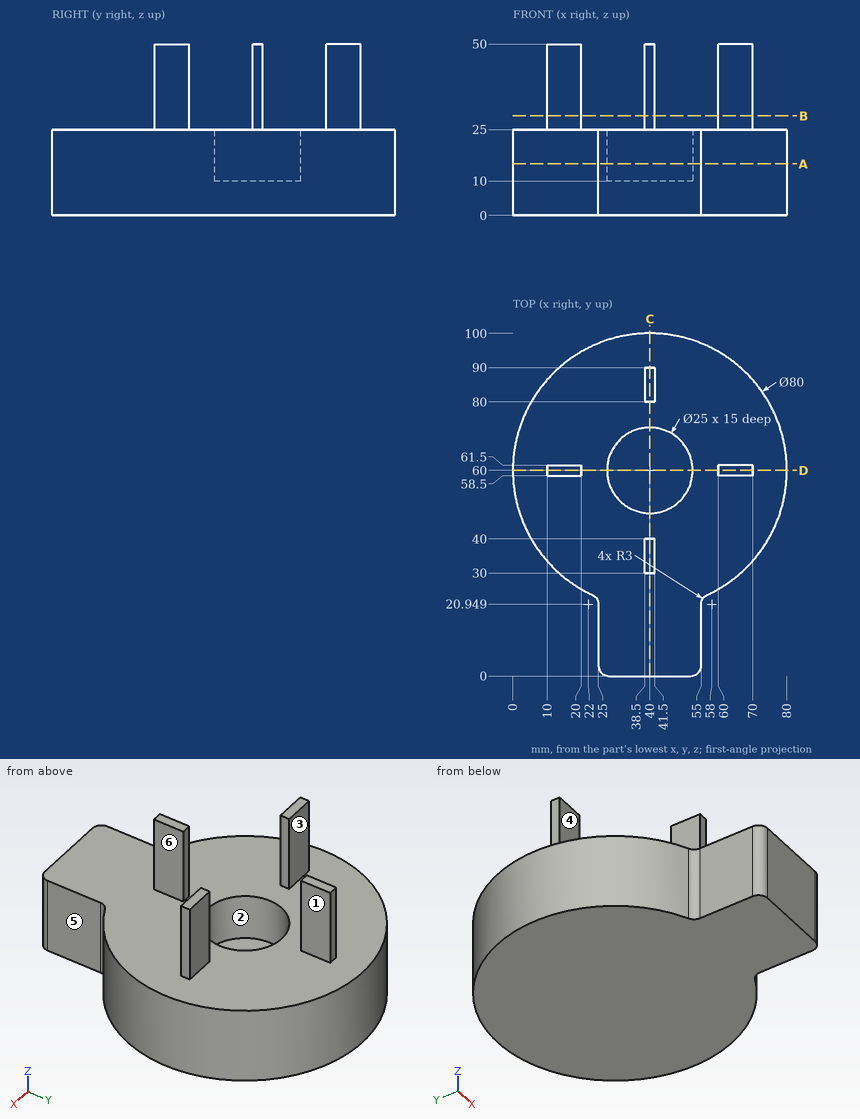
Answer from the drawing. Dimensions are ordinates in mm from the lowest x, y and z of the part. A direction names the side the tool comes from. Give positions to 0.01 mm unless a question says otherwise; leave off trailing zeros. Order: outer loops, then holes, each group sorted by start corner. A loop starts at its lowest first (then second) coordinate and runs counter-clockwise, first axis right, second up. Notation, with made-up numbers: (8, 3) - (30, 3) arc R6 cw to (30, 7) - close; hole circle Ø7 at (-26, 12). An arc over 180 degrees is marked (long way). One line per item, written item: value. Start each with the question number.
1) Find the intervals of material crossed by L1, parallel to Y at x = 40, z = 13; L2, parallel to Z at x = 21.5, y = 44.5; L3, parallel to X at y = 13, z = 21.5, in increasing order.
2) The mould has two halves that part along Y. Classify the marked faces 1, 2 and 3: released by +Y, released by -Y, zero draft, split by the parting line, or undercut.
3) A cutting plane is placed at C-C on x = 40. Give the vertices of the cut face in (y, z), then the cut area to 4 significant figures.
4) A cutting plane is placed at B-B on z = 29. Give the vertices of the cut face in (x, y).
5) A cutting plane is placed at A-A on z = 15. Give the vertices of the cut face in (x, y).
6) A cutting plane is placed at D-D on y = 60. Give the vertices of the cut face in (x, z), then the cut area to 4 significant figures.
7) A tool of negligible diameter and unlimited length cuts with its end or side. For the marked faces 4, 5 and 6, from which of +Z, -Z, +X, -X, +Y, -Y can it reach the whole face along a straight path? Write none if from no direction.
8) Given pin 1 Ø1 at (x, z) = (16.5, 18) entering from +Y; pin 2 Ø8 at (x, z) = (65.5, 34.5) entering from -Y; pin 3 Ø8 at (y, z) = (83, 33) entering from +X, each flat-ended and moving along its own axis, determine where each tip first touches the part or whether it passes through.
Answer sheet:
1. L1: y = 0 to 47.5, 72.5 to 100
1. L2: z = 0 to 25
1. L3: x = 25 to 55
2. face 1: zero draft
2. face 2: undercut
2. face 3: released by +Y
3. outline: (0, 0) - (100, 0) - (100, 25) - (90, 25) - (90, 50) - (80, 50) - (80, 25) - (72.5, 25) - (72.5, 10) - (47.5, 10) - (47.5, 25) - (40, 25) - (40, 50) - (30, 50) - (30, 25) - (0, 25) - close
3. area: 2,625 mm2
4. outline: (10, 58.5) - (20, 58.5) - (20, 61.5) - (10, 61.5) - close; (38.5, 30) - (41.5, 30) - (41.5, 40) - (38.5, 40) - close; (38.5, 80) - (41.5, 80) - (41.5, 90) - (38.5, 90) - close; (60, 58.5) - (70, 58.5) - (70, 61.5) - (60, 61.5) - close
5. outline: (23.26, 23.67) arc R3 cw to (25, 20.95) - (25, 3) arc R3 ccw to (28, 0) - (52, 0) arc R3 ccw to (55, 3) - (55, 20.95) arc R3 cw to (56.74, 23.67) arc R40 ccw (long way) to start; hole circle Ø25 at (40, 60)
6. outline: (0, 0) - (80, 0) - (80, 25) - (70, 25) - (70, 50) - (60, 50) - (60, 25) - (52.5, 25) - (52.5, 10) - (27.5, 10) - (27.5, 25) - (20, 25) - (20, 50) - (10, 50) - (10, 25) - (0, 25) - close
6. area: 2,125 mm2
7. face 4: +Z, +X, -X, -Y
7. face 5: +Z, -Z, +X, -Y
7. face 6: +Z, +X, +Y, -Y
8. pin 1: stops at y = 92.73
8. pin 2: stops at y = 58.5
8. pin 3: stops at x = 41.5
